```python
from build123d import *

# Parameters (mm, degrees)
F1_W     = 94
F1_H     = 34
F2_DEPTH = 600


with BuildPart() as f2:
    # F1 (on Right) → F2 (new body, symmetric)
    with BuildSketch(Plane.YZ):
        with BuildLine():
            ThreePointArc((-19.2521204937, -49.7380952381), (-18.6663340561, -51.1523088005), (-17.2521204937, -51.7380952381))
            Line((-17.2521204937, -51.7380952381), (78.7478795063, -51.7380952381))
            ThreePointArc((78.7478795063, -51.7380952381), (80.1620930687, -51.1523088005), (80.7478795063, -49.7380952381))
            Line((80.7478795063, -49.7380952381), (80.7478795063, -13.7380952381))
            ThreePointArc((80.7478795063, -13.7380952381), (80.1620930687, -12.3238816757), (78.7478795063, -11.7380952381))
            Line((78.7478795063, -11.7380952381), (-17.2521204937, -11.7380952381))
            ThreePointArc((-17.2521204937, -11.7380952381), (-18.6663340561, -12.3238816757), (-19.2521204937, -13.7380952381))
            Line((-19.2521204937, -13.7380952381), (-19.2521204937, -49.7380952381))
        make_face()
        with Locations((30.7478795063, -31.7380952381)):
            Rectangle(F1_W, F1_H, mode=Mode.SUBTRACT)
    extrude(amount=F2_DEPTH, both=True)


with BuildPart() as f3_1:
    # F3: copy of F2
    add(f2.part)


solid = f2.part
```
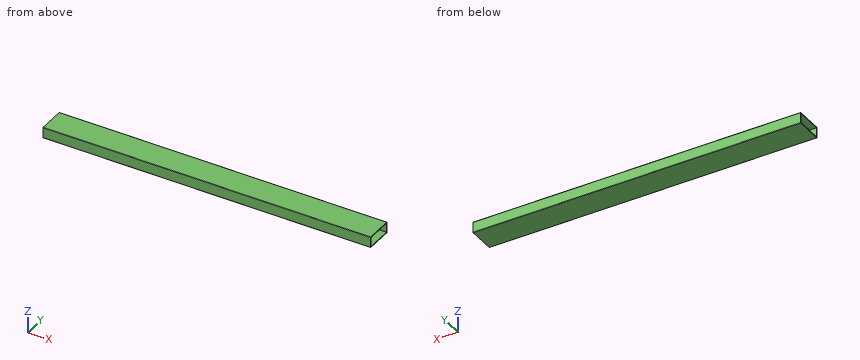
Could you check a few things on this model? Use its own coordinates, in mm. Round coordinates to 2 decimals unless told otherwise and drop trailing zeros. Loops run counter-clockwise (first coordinate to the right, second up) from the corner with the lowest first, then second, coordinate; pieces in that order, holes last.
Q1. I want a section at C-C (x = -249.5). Write out the boundary of the cut face in (y, z), and give its area (3 significant figures).
Q2. I want a section at A-A (y = 27.5). Write out the boundary of the cut face in (x, z).
Q3. I want a section at B-B (z = -36). Write out the boundary of the cut face in (x, y), and give its area (3 significant figures).
Q4. Please list where these lines run through material, in increasing order: L1, parallel to Y at x = -66, z = -42.5; L2, parallel to Z at x = 143, y = -8; L3, parallel to Y at x = 533, z = -50.
Answer below:
1. outline: (-19.25, -49.74) arc R2 ccw to (-17.25, -51.74) - (78.75, -51.74) arc R2 ccw to (80.75, -49.74) - (80.75, -13.74) arc R2 ccw to (78.75, -11.74) - (-17.25, -11.74) arc R2 ccw to (-19.25, -13.74) - close; hole (-16.25, -48.74) - (77.75, -48.74) - (77.75, -14.74) - (-16.25, -14.74) - close
1. area: 801 mm2
2. outline: (-600, -51.74) - (600, -51.74) - (600, -48.74) - (-600, -48.74) - close; (-600, -14.74) - (600, -14.74) - (600, -11.74) - (-600, -11.74) - close
3. outline: (-600, -19.25) - (600, -19.25) - (600, -16.25) - (-600, -16.25) - close; (-600, 77.75) - (600, 77.75) - (600, 80.75) - (-600, 80.75) - close
3. area: 7,200 mm2
4. L1: y = -19.25 to -16.25, 77.75 to 80.75
4. L2: z = -51.74 to -48.74, -14.74 to -11.74
4. L3: y = -19.23 to 80.73
